from build123d import *

# Parameters (mm, degrees)
F3_R     = 3.175
F4_DEPTH = 25.4


with BuildPart() as f2:
    # F0 (on Front) → F2 (revolve)
    with BuildSketch(Plane.XZ):
        with BuildLine():
            Line((0, -9.525), (0, 9.525))
            ThreePointArc((0, 9.525), (-9.525, 0), (0, -9.525))
        make_face()
    revolve(axis=Axis((0, 0, 0), (0, 0, 1)))


with BuildPart() as f4:
    # F3 (on Front) → F4 (new body)
    with BuildSketch(Plane.XZ):
        Circle(F3_R)
    extrude(amount=F4_DEPTH)


with BuildPart() as f2_1:
    add(f2.part)

    # F5: cut F4
    add(f4.part, mode=Mode.SUBTRACT)


solid = f2_1.part
For this review, take the finished solid that the model builds, in its own axes (mm). Round coordinates to 2 decimals unless told otherwise and drop trailing zeros. Write each loop counter-clockwise with the first axis right and the second up, starting at its lowest first coordinate (ties: lowest second). Pieces come first, ordered by that corner, then holes. Notation, with made-up numbers: (-37, 88.5) - (-16, 88.5) arc R14 ccw to (-16, 102.5) - close; hole circle Ø8 at (20.5, 21.25). An arc over 180 degrees is marked (long way). Write item = value, one per line. Start each with the question number.
1. Consider section D-D on y = 5.5. State the section outline as (x, z) points, plus the area to 3 significant figures.
2. Consider section C-C on z = 0. State the section outline as (x, y) points (3 decimals).
3. Consider section A-A on x = 0. State the section outline as (y, z) points (3 decimals).
4. Wall thickness on L1, parallel to Z at x = 0, y = -1.75 (3 decimals); L2, parallel to Y at x = -0.25, z = 0; L3, parallel to X at y = -5.5, z = 0 (3 decimals): over which ranges is each line inside the solid? List them lowest first.
5. Draft analysis for pull direction Z (two halves, no side actions). For faces 1 (the face through (-0.69, -4.43, -3.1)), 2 (the face through (0, 0, 0)), state which applies: released by +Z, released by -Z, zero draft, split by the parting line, or undercut.
6. For pin 1 Ø8 at (y, z) = (7, -6.5) entering from -X; pin 2 Ø5 at (x, y) = (5.5, 4) entering from +Z; pin 3 Ø10 at (x, z) = (6.5, -2.5) entering from -Y, all flat-tipped, find the tip position at first contact; note any pin that passes through.
7. Consider section B-B on y = -0.5. State the section outline as (x, z) points (3 decimals), plus the area to 3 significant figures.
Evaluation:
q1.outline = circle Ø15.55 at (0, 0)
q1.area = 190 mm2
q2.outline = (-3.175, -8.98) - (-3.175, 0) - (3.175, 0) - (3.175, -8.98) arc R9.525 ccw (long way) to start
q3.outline = (-8.98, -3.175) arc R9.525 ccw (long way) to (-8.98, 3.175) - (0, 3.175) - (0, -3.175) - close
q4.L1 = -9.363 to -3.175, 3.175 to 9.363
q4.L2 = 0 to 9.52
q4.L3 = -7.777 to -3.175, 3.175 to 7.777
q5.face_1 = undercut
q5.face_2 = undercut
q6.pin_1 = -7.74
q6.pin_2 = 8.5
q6.pin_3 = -8.98
q7.outline = circle Ø19.024 at (0, 0); hole circle Ø6.35 at (0, 0)
q7.area = 253 mm2
